The model under review builds one solid part; all positions refer to its coordinate system, in mm. Face numbers are marked on the shaded views. A direction names the side the tool comes from. Give positions to 0.01 mm unless a question says otherwise; leave off trailing zeros. Loops run counter-clockwise (first coordinate to the right, second up) from the corner with the lowest first, then second, coordinate; pieces in that order, holes last. Notation, with made-up numbers: M 23,38.25 L 30,38.25 A22 ccw 30,62.25 Z; hole C -23,-28 d2. An arc over 180 degrees is marked long. Return JSON: item names as keys, results as strings.
```python
from build123d import *

# Parameters (mm, degrees)
BOSS_EXTRUDE1_DEPTH    = 7.5
CUT_EXTRUDE1_DEPTH     = 5
M4_CLEARANCE_HOLE1_D   = 4.5
BOSS_EXTRUDE2_DEPTH    = 15
CUT_EXTRUDE5_START     = -15
CUT_EXTRUDE5_DEPTH     = 5
FILLET8_R              = 1
FILLET4_R              = 19
FILLET1_R              = 0.5
FILLET7_R              = 5
FILLET6_RADIUS         = 5
FILLET6_LENGTH         = 8.210867904
F_10_CLEARANCE_HOLE1_D = 5.1054
FILLET9_R              = 5
FILLET10_R             = 1
SKETCH15_R             = 6
CUT_EXTRUDE7_DEPTH     = 16


with BuildPart() as part:
    # Sketch1 → Boss-Extrude1 (new, symmetric)
    with BuildSketch(Plane.XY):
        with BuildLine():
            Line((-6.749999988, 53.250000012), (6.749999988, 53.250000012))
            Line((6.749999988, 53.250000012), (6.749999988, 0))
            ThreePointArc((6.749999988, 0), (0, -6.749999988), (-6.749999988, 0))
            Line((-6.749999988, 0), (-6.749999988, 53.250000012))
        make_face()
    extrude(amount=BOSS_EXTRUDE1_DEPTH, both=True)

    # Sketch3 → Cut-Extrude1 (cut)
    with BuildSketch(Plane.XY.offset(7.5)):
        with BuildLine():
            Line((-6.749999988, 0), (-6.749999988, 8.205771407))
            Line((-6.749999988, 8.205771407), (-2.249999988, 9.411542773))
            Line((-2.249999988, 9.411542773), (6.749999988, 25))
            Line((6.749999988, 25), (6.749999988, 0))
            ThreePointArc((6.749999988, 0), (0, -6.749999988), (-6.749999988, 0))
        make_face()
    cut_extrude1 = extrude(amount=-CUT_EXTRUDE1_DEPTH, mode=Mode.SUBTRACT)

    # M4 Clearance Hole1 (through all)
    with Locations(Plane.XY.offset(2.5)):
        with Locations((0, 0)):
            Hole(M4_CLEARANCE_HOLE1_D / 2)

    # Mirror1: Cut-Extrude1 across plane
    add(cut_extrude1.mirror(Plane.XY), mode=Mode.SUBTRACT)

    # Sketch8 → Boss-Extrude2 (add)
    with BuildSketch(Plane.XY.offset(7.5)):
        Polygon((13.103097639, 64.300161569), (8.404634535, 62.590060852), (-6.749999988, 57.074224974), (-6.749999988, 53.250000012), (6.749999988, 53.250000012), (15.911379857, 56.584469589), align=None)
    extrude(amount=-BOSS_EXTRUDE2_DEPTH)

    # Sketch9 → Cut-Extrude5 (cut)
    with BuildSketch(Plane.XY.offset(7.5).offset(CUT_EXTRUDE5_START)):
        Polygon((-6.749999988, 16.617314139), (2.708548104, 33), (6.749999988, 33), (6.749999988, 53.250000012), (15.911379857, 56.584469589), (13.103097639, 64.300161569), (-6.749999988, 57.074224974), align=None)
    extrude(amount=CUT_EXTRUDE5_DEPTH, mode=Mode.SUBTRACT)

    # Fillet8
    fillet8_edges = [part.edges().sort_by_distance(p)[0] for p in [
        (2.708548104, 33, -5),
    ]]
    fillet(fillet8_edges, radius=FILLET8_R)

    # Fillet4
    # the kernel refuses this fillet: 19 mm, written as the material it adds along each edge
    with BuildSketch(Plane(origin=(3.285898373, 33, -2.5), x_dir=(0, 1, 0), z_dir=(1, 0, 0))) as fillet4_piece_1:
        with BuildLine():
            CenterArc((12.845232579, -19), FILLET4_R, 90, 42.536898363)
            Line((0, -5), (0, 0))
            Line((0, 0), (12.845232579, 0))
        make_face()
    extrude(amount=3.464101615)
    with BuildSketch(Plane(origin=(-22.806540711, -11.193430188, -2.5), x_dir=(-0.8660254037844388, 0.4999999999999999, 0), z_dir=(0.4999999999999999, 0.8660254037844388, 0))) as fillet4_piece_2_section:
        with BuildLine():
            CenterArc((12.845232579, -19), FILLET4_R, 90, 42.536898363)
            Line((0, -5), (0, 0))
            Line((0, 0), (12.845232579, 0))
        make_face()
    fillet4_piece_2 = extrude(amount=50.452827361, mode=Mode.PRIVATE)
    fillet4_piece_2 = split(fillet4_piece_2, bisect_by=Plane(origin=(-6.749999988, -11.193430188, -2.5), z_dir=(1, 0, 0)), keep=Keep.TOP, mode=Mode.PRIVATE)
    add(fillet4_piece_2)
    with BuildSketch(Plane(origin=(3.285898373, 32, -2.5), x_dir=(-0.8660254037844386, 0.4999999999999999, 0), z_dir=(-0.4999999999999999, -0.8660254037844386, 0))) as fillet4_piece_3_section:
        with BuildLine():
            CenterArc((13.845232579, 19), FILLET4_R, 227.463101637, 42.536898363)
            Line((1, 5), (1, 0))
            Line((1, 0), (13.845232579, 0))
        make_face()
    fillet4_piece_3 = revolve(axis=Axis((3.285898373, 32, -2.5), (0, 0, -1)), revolution_arc=60, mode=Mode.PRIVATE)
    fillet4_piece_3 = split(fillet4_piece_3, bisect_by=Plane(origin=(-6.749999988, 32, -2.5), z_dir=(1, 0, 0)), keep=Keep.TOP, mode=Mode.PRIVATE)
    add(fillet4_piece_3)

    # Fillet1
    fillet1_edges = [part.edges().sort_by_distance(p)[0] for p in [
        (-6.749999988, 8.205771407, 5),
        (-6.749999988, 8.205771407, -5),
    ]]
    fillet(fillet1_edges, radius=FILLET1_R)

    # Fillet7
    fillet7_edges = [part.edges().sort_by_distance(p)[0] for p in [
        (6.749999988, 25, 5),
        (6.749999988, 25, -5),
    ]]
    fillet(fillet7_edges, radius=FILLET7_R)

    # Fillet6: full round fillet: the end face becomes a half cylinder, R = half its width
    fillet6_face = Plane((14.507238748, 60.442315579, 2.5), x_dir=(0.342020143326, -0.939692620786, 0), z_dir=(0.939692620786, 0.342020143326, 0))  # on the end face: x along it, z out of the body
    fillet6_slab = fillet6_face.offset(-FILLET6_RADIUS / 2) * Box(FILLET6_LENGTH, 2 * FILLET6_RADIUS, FILLET6_RADIUS, mode=Mode.PRIVATE)  # the body's end, R deep
    fillet6_round = Plane((9.808775644, 58.732214862, 2.5), x_dir=(0.939692620786, 0.342020143326, 0), z_dir=(0.342020143326, -0.939692620786, 0)) * Cylinder(FILLET6_RADIUS, FILLET6_LENGTH, mode=Mode.PRIVATE)  # its axis R under the face
    add(fillet6_slab - fillet6_round, mode=Mode.SUBTRACT)

    # #10 Clearance Hole1 (through all)
    with Locations(Plane(origin=(-19.132902326, 52.56721711, 0), x_dir=(0.9396926207859103, 0.3420201433256639, 0), z_dir=(-0.3420201433256639, 0.9396926207859103, 0))):
        with Locations((29.304834637, -2.5)):
            Hole(F_10_CLEARANCE_HOLE1_D / 2)

    # Fillet9
    fillet9_edges = [part.edges().sort_by_distance(p)[0] for p in [
        (-2.249999988, 9.411542773, 5),
        (-2.249999988, 9.411542773, -5),
    ]]
    fillet(fillet9_edges, radius=FILLET9_R)

    # Fillet10
    fillet10_edges = [part.edges().sort_by_distance(p)[0] for p in [
        (6.749999988, 53.250000012, 2.5),
    ]]
    fillet(fillet10_edges, radius=FILLET10_R)

    # Sketch15 → Cut-Extrude7 (cut)
    with BuildSketch(Plane(origin=(-16.324620109, 44.85152513, 0), x_dir=(0.9396926207859103, 0.3420201433256634, 0), z_dir=(0.3420201433256634, -0.9396926207859103, 0))):
        with Locations((29.304834637, 2.5)):
            Circle(SKETCH15_R)
    extrude(amount=CUT_EXTRUDE7_DEPTH, mode=Mode.SUBTRACT)


solid = part.part
```
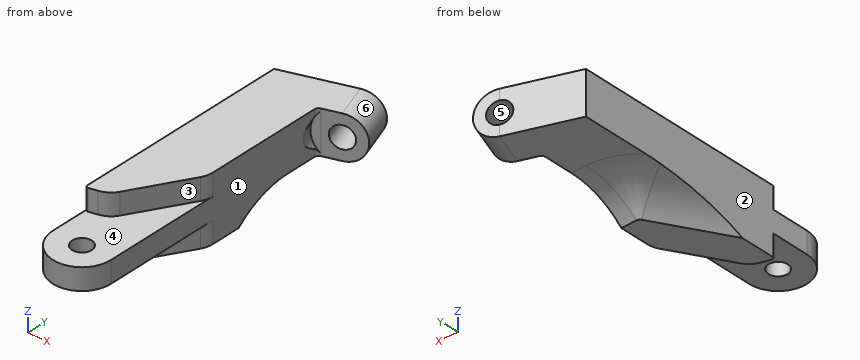
1) Insertion check: pin 1 (1.5 mm diameter, centred on y = 38, z = 0.5, fed in from +X); pin 2 (2 mm diameter, centred on x = 2.5, z = 0, fed in from -Y); pin 3 (3.5 mm diameter, centred on x = 0, y = 0, fed in from +Z); pin 4 (8 mm diameter, centred on x = 3.5, z = 5, fed in from +Y). Each pin has a flat end and moves straight along its axis. Give the tip position at first contact, or say it passes through.
From the geometry:
{"pin 1": "x = 6.75", "pin 2": "y = -6.58", "pin 3": "through", "pin 4": "y = 62.26"}
2) Consider section C-C on y = 48.5. Write out the cut boundary in (x, z), then the cut area to 3 significant figures.
From the geometry:
{"outline": "M -6.75,-2.5 L 6.75,-2.5 L 6.75,7.5 L -6.75,7.5 Z", "area": "135 mm²"}
3) Consider section B-B on z = 4. Write out the cut boundary in (x, y).
From the geometry:
{"outline": "M -6.75,8.86 A0.5 ccw -6.12,8.37 L -4.25,8.88 A5 ccw -1.21,11.21 L 6.08,23.84 A5 ccw 6.75,26.34 L 6.75,50.15 L 5.75,52.89 L 9.27,54.17 L 6.46,61.88 L -6.75,57.07 Z; M 10.35,63.3 L 13.15,55.58 L 15.69,56.51 L 12.89,64.22 Z"}
4) Wall thickness on L1, parallel to X at y = 38.5, z = -1; L2, parallel to Z at x = 1, y = 13.5; L3, parallel to Z at x = 3, y = 50: over which ranges is each line inside the solid? List them lowest first. Write a range as from..to.
From the geometry:
{"L1": "-6.75..6.75", "L2": "-2.5..2.5", "L3": "-2.5..7.5"}
5) The part is to be moulded in two halves that separate along Y. For the marked faces 4, 5 and 6, say which applies: released by +Y, released by -Y, zero draft, split by the parting line, or undercut.
From the geometry:
{"face 4": "zero draft", "face 5": "undercut", "face 6": "released by +Y"}
6) Tool access review of the marked faces 1, 2 and 3: name each direction out of +Z, -Z, +X, -X, +Y, -Y from which nothing blocks a thin tool from reaching the whole face with its end or side.
From the geometry:
{"face 1": "+Z, -Z, +X, -Y", "face 2": "+Z, -Z, -X, +Y, -Y", "face 3": "+Z, +X, -Y"}
7) Consider section A-A on z = 1. Write out the cut boundary in (x, y), then the cut area to 3 significant figures.
From the geometry:
{"outline": "M -6.75,0 A6.75 ccw 6.75,0 L 6.75,50.15 L 5.75,52.89 L 9.27,54.17 L 6.46,61.88 L -6.75,57.07 Z; M 10.35,63.3 L 13.15,55.58 L 15.69,56.51 L 12.89,64.22 Z; hole C 0,0 d4.5", "area": "890 mm²"}
